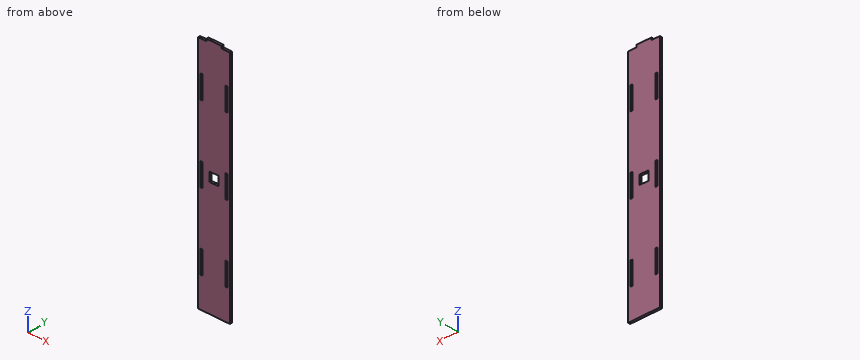
```python
from build123d import *

# Parameters (mm, degrees)
SKETCH1_W           = 3
SKETCH1_H           = 30
SKETCH1_W_2         = 12
SKETCH1_H_2         = 12
BOSS_EXTRUDE1_DEPTH = 3


with BuildPart() as part:
    # Sketch1 → Boss-Extrude1 (new body)
    with BuildSketch(Plane(origin=(0, 0, 0), x_dir=(1, 0, 0), z_dir=(0, 1, 0))):
        Polygon((31, 0), (42, 0), (42, 310), (0, 310), (0, 0), (11, 0), (11, -3), (31, -3), align=None)
        with Locations((37.5, 55)):
            Rectangle(SKETCH1_W, SKETCH1_H, mode=Mode.SUBTRACT)
        with Locations((37.5, 155)):
            Rectangle(SKETCH1_W, SKETCH1_H, mode=Mode.SUBTRACT)
        with Locations((37.5, 255)):
            Rectangle(SKETCH1_W, SKETCH1_H, mode=Mode.SUBTRACT)
        with Locations((4.5, 255)):
            Rectangle(SKETCH1_W, SKETCH1_H, mode=Mode.SUBTRACT)
        with Locations((4.5, 155)):
            Rectangle(SKETCH1_W, SKETCH1_H, mode=Mode.SUBTRACT)
        with Locations((4.5, 55)):
            Rectangle(SKETCH1_W, SKETCH1_H, mode=Mode.SUBTRACT)
        with Locations((21, 153)):
            Rectangle(SKETCH1_W_2, SKETCH1_H_2, mode=Mode.SUBTRACT)
    extrude(amount=BOSS_EXTRUDE1_DEPTH)


solid = part.part
```
Work out the finished part from the listing and answer in its coordinate system (mm). Round coordinates to 2 decimals unless told otherwise and drop trailing zeros. Loops run counter-clockwise (first coordinate to the right, second up) from the corner with the lowest first, then second, coordinate; pieces in that order, holes last. Notation, with made-up numbers: M 28,14 L 82,14 A19 ccw 82,30 Z; hole C -14.5,-29.5 d1. An arc over 180 degrees is marked long. One line per question, with ' | ' between items.
Q1. Find section C-C, the plane y = 1.1. State how many separate pieces and enclosed holes the cut face has, then the cut area to 3 significant figures.
Conclusion:
separate pieces: 1 | enclosed holes: 7 | area: 12,400 mm2
Q2. Each of these flat-tipped pins is pushed along its axis until it touches: pin 1 Ø6 at (x, z) = (18, -170) entering from -Y; pin 2 Ø1.5 at (x, y) = (4, 1.5) entering from +Z. Where does it stop, or does it pass through?
Conclusion:
pin 1: stops at y = 0 | pin 2: stops at z = 0
Q3. Find section A-A, the plane z = -45. Give the vertices of the cut face in (x, y), then the cut area to 3 significant figures.
Conclusion:
outline: M 0,0 L 3,0 L 3,3 L 0,3 Z; M 6,0 L 36,0 L 36,3 L 6,3 Z; M 39,0 L 42,0 L 42,3 L 39,3 Z | area: 108 mm2
Q4. Consider line 1 along Z through (x, y) = (4, 0.85); line 2 along X through (y, z) = (0.1, -157.5); line 3 along X through (y, z) = (2.15, -65). Determine where each line is inside the solid, lowest interval first. Write a range as from..to.
Conclusion:
line 1: z = -310..-270, -240..-170, -140..-70, -40..0 | line 2: x = 0..3, 6..15, 27..36, 39..42 | line 3: x = 0..3, 6..36, 39..42
Q5. Find section B-B, the plane x = 21. Give the vertices of the cut face in (y, z).
Conclusion:
outline: M 0,-310 L 3,-310 L 3,-159 L 0,-159 Z; M 0,-147 L 3,-147 L 3,3 L 0,3 Z
